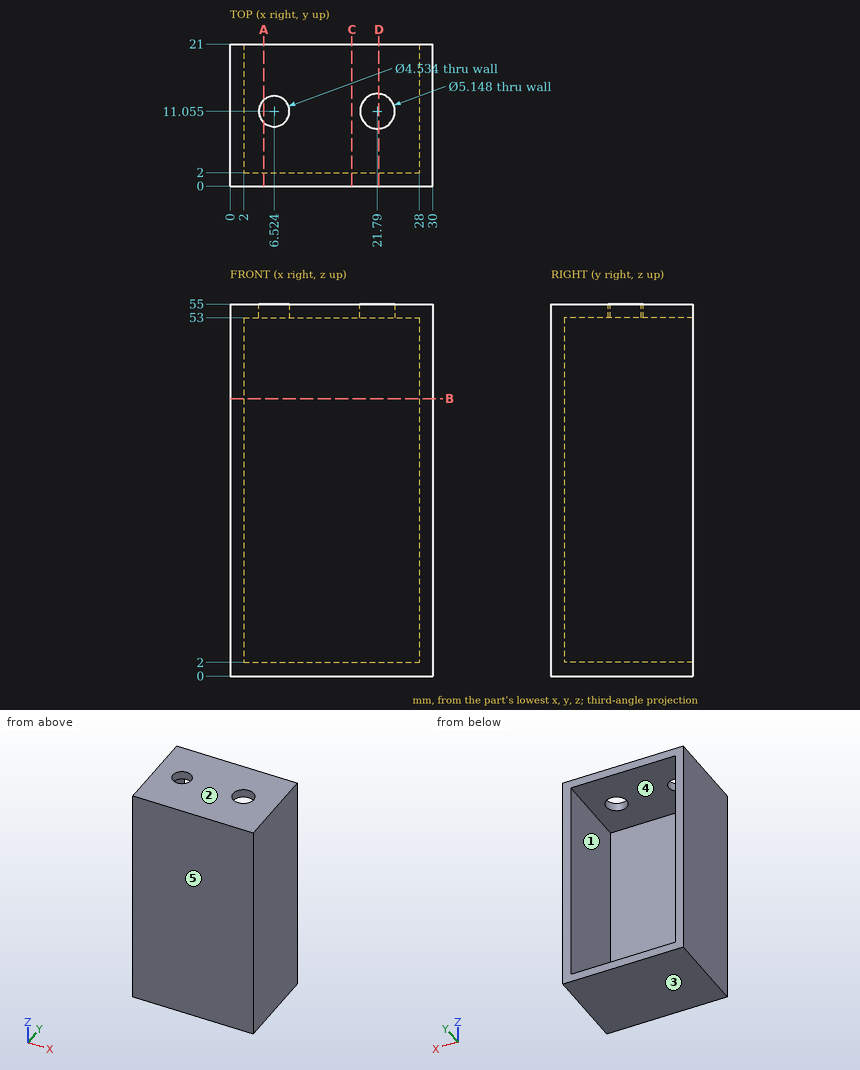
For this review, use the dimensioned drawing (mm, ordinates from the lowest corner) and the shaded views. A direction names the side the tool comes from. Coordinates: 2 decimals unless noted, no trailing zeros. Loops run counter-clockwise (first coordinate to the right, second up) from the corner with the lowest first, then second, coordinate; pieces in that order, holes last. Notation, with made-up numbers: (6.25, 74.25) -> (63.25, 74.25) arc R27 cw to (63.25, 108.25) -> close; hole circle Ø11 at (36, 69.25). An arc over 180 degrees is marked (long way). Use a Markdown table: item, result. Add a question column.
1. To check wall thickness, follow line 1 (Z direction, x = 25.25, y = 19.75); line 2 (X direction, y = 10.25, z = 47); line 3 (Y direction, x = 6.5, z = 33). State the ranges of each line that lie inside material, in increasing order.
2. Machinability: for the marked faces 4 and 5, which of the approach directions +Z, -Z, +X, -X, +Y, -Y give a long, thin tool a straight path to every point of the face, cutting with its end or side? Answer none if there is none.
3. Draft analysis for pull direction Z (two halves, no side actions). For the marked faces 1, 2 and 3, state which applies: pulls with the +Z half, pulls with the -Z half, needs draft (parallel to the pull), parting line crosses it, or undercut.
4. Add section B-B on z = 41. Write out the cut boundary in (x, y).
5. Clearance check with flat-ended pins moving along their axes: pin 1 Ø13 at (x, z) = (9.5, 19) entering from +Y; pin 2 Ø3.5 at (x, y) = (6.52, 11.05) entering from +Z. State where each tip first meets the part, or that it passes through.
6. Add section D-D on x = 22. Write out the cut boundary in (y, z).
7. Add section A-A on x = 5. Write out the cut boundary in (y, z).
8. Add section C-C on x = 18. Write out the cut boundary in (y, z), plus the area to 3 significant figures.
Returned:
| question | item | result |
|---|---|---|
| 1 | line 1 | z = 0 to 2, 53 to 55 |
| 1 | line 2 | x = 0 to 2, 28 to 30 |
| 1 | line 3 | y = 0 to 2 |
| 2 | face 4 | +Y |
| 2 | face 5 | +Z, -Z, +X, -X, -Y |
| 3 | face 1 | undercut |
| 3 | face 2 | pulls with the +Z half |
| 3 | face 3 | pulls with the -Z half |
| 4 | outline | (0, 0) -> (30, 0) -> (30, 21) -> (28, 21) -> (28, 2) -> (2, 2) -> (2, 21) -> (0, 21) -> close |
| 5 | pin 1 | stops at y = 2 |
| 5 | pin 2 | stops at z = 2 |
| 6 | outline | (0, 0) -> (21, 0) -> (21, 2) -> (2, 2) -> (2, 53) -> (8.49, 53) -> (8.49, 55) -> (0, 55) -> close; (13.62, 53) -> (21, 53) -> (21, 55) -> (13.62, 55) -> close |
| 7 | outline | (0, 0) -> (21, 0) -> (21, 2) -> (2, 2) -> (2, 53) -> (9.38, 53) -> (9.38, 55) -> (0, 55) -> close; (12.73, 53) -> (21, 53) -> (21, 55) -> (12.73, 55) -> close |
| 8 | outline | (0, 0) -> (21, 0) -> (21, 2) -> (2, 2) -> (2, 53) -> (21, 53) -> (21, 55) -> (0, 55) -> close |
| 8 | area | 186 mm² |
